from build123d import *

# Parameters (mm, degrees)
SKETCH2_W           = 3.765548925
SKETCH2_H           = 14.748929387
SKETCH2_W_2         = 4.619974481
CUT_EXTRUDE1_DEPTH  = 17.5
CHAMFER1_SIZE       = 0.353571801
CHAMFER1_SIZE_2     = 0.5
SKETCH3_R           = 3
CUT_EXTRUDE2_DEPTH  = 35
SKETCH4_R           = 3.5
SKETCH4_R_2         = 3
BOSS_EXTRUDE1_DEPTH = 15
BOSS_EXTRUDE2_DEPTH = 1
BOSS_EXTRUDE3_START = -1
SKETCH4_2_R         = 3.5
SKETCH4_2_R_2       = 3
BOSS_EXTRUDE3_DEPTH = 1
BOSS_EXTRUDE4_START = -1
BOSS_EXTRUDE4_DEPTH = 1
FILLET1_R           = 1
FILLET2_R           = 10


# Some blends are built 0.0001 mm under size
with BuildPart() as part:
    # Sketch1 → Revolve1 (revolve)
    with BuildSketch(Plane(origin=(0, 0, 0), x_dir=(0, 0, -1), z_dir=(1, 0, 0))):
        with BuildLine():
            Line((0, 3.5), (0, 0))
            Line((0, 0), (4.5, 0))
            ThreePointArc((4.5, 0), (8, 3.5), (11.5, 0))
            Line((11.5, 0), (14, 0))
            ThreePointArc((14, 0), (11.451186904, 4.908086078), (5.97023035, 5.6462408))
            Line((5.97023035, 5.6462408), (0, 3.5))
        make_face()
    revolve(axis=Axis((0, 0, 0), (0, 0, -1)))

    # Sketch2 → Cut-Extrude1 (cut, symmetric)
    with BuildSketch(Plane(origin=(0, 0, 0), x_dir=(1, 0, 0), z_dir=(0, 1, 0))):
        with Locations((-4.382774463, 6.625535306)):
            Rectangle(SKETCH2_W, SKETCH2_H)
        with Locations((4.80998724, 6.625535306)):
            Rectangle(SKETCH2_W_2, SKETCH2_H)
    extrude(amount=CUT_EXTRUDE1_DEPTH, both=True, mode=Mode.SUBTRACT)

    # Chamfer1
    # the kernel refuses this chamfer: 0.5, 0.353571801 mm, written as the material it takes off along each edge
    with BuildSketch(Plane(origin=(-2.5, 0, -8), x_dir=(0, 0, 1), z_dir=(0, 1, 0))) as chamfer1_piece_1:
        with BuildLine():
            Line((2.807242504, 0.409691525), (2.449489743 + CHAMFER1_SIZE * 0.999999998636, 0))
            Line((2.449489743 + CHAMFER1_SIZE * 0.999999998636, 0), (2.449489743, 0))
            ThreePointArc((2.449489743, 0), (2.641353047, 0.203643303), (2.807242504, 0.409691525))
        make_face()
    revolve(axis=Axis((-2.5, 0, -8), (1, 0, 0)), mode=Mode.SUBTRACT)
    with BuildSketch(Plane(origin=(2.5, 0, -8), x_dir=(0, 0, -1), z_dir=(0, 1, 0))) as chamfer1_piece_2:
        with BuildLine():
            Line((2.449489743 + CHAMFER1_SIZE_2, 0), (2.689392867, 0.260096876))
            ThreePointArc((2.689392867, 0.260096876), (2.573005025, 0.127312675), (2.449489743, 0))
            Line((2.449489743, 0), (2.449489743 + CHAMFER1_SIZE_2, 0))
        make_face()
    revolve(axis=Axis((2.5, 0, -8), (-1, 0, 0)), mode=Mode.SUBTRACT)

    # Sketch3 → Cut-Extrude2 (cut)
    with BuildSketch(Plane(origin=(2.5, 0, 0), x_dir=(0, 0, -1), z_dir=(1, 0, 0))):
        with Locations((8, 0)):
            Circle(SKETCH3_R)
    extrude(amount=-CUT_EXTRUDE2_DEPTH, mode=Mode.SUBTRACT)

    # Sketch4 → Boss-Extrude1 (add)
    with BuildSketch(Plane.XY):
        with Locations(Location((0, 0, 0), (0, 0, 135.584691403))):
            Circle(SKETCH4_R)
        with Locations(Location((0, 0, 0), (0, 0, 213.557309762))):
            Circle(SKETCH4_R_2, mode=Mode.SUBTRACT)
    extrude(amount=BOSS_EXTRUDE1_DEPTH)

    # Sketch5 → Boss-Extrude2 (add)
    with BuildSketch(Plane.XY):
        with BuildLine():
            Line((2.5, 1.658312395), (2.5, -1.658312395))
            ThreePointArc((2.5, -1.658312395), (2.872281323, -0.866025404), (3, 0))
            ThreePointArc((3, 0), (2.872281323, 0.866025404), (2.5, 1.658312395))
        make_face()
        with BuildLine():
            ThreePointArc((-2.5, -1.658312395), (0, -3), (2.5, -1.658312395))
            Line((2.5, -1.658312395), (2.5, 1.658312395))
            ThreePointArc((2.5, 1.658312395), (0, 3), (-2.5, 1.658312395))
            Line((-2.5, 1.658312395), (-2.5, -1.658312395))
        make_face()
        with BuildLine():
            ThreePointArc((-2.5, 1.658312395), (-3, 0), (-2.5, -1.658312395))
            Line((-2.5, -1.658312395), (-2.5, 1.658312395))
        make_face()
    extrude(amount=BOSS_EXTRUDE2_DEPTH)

    # Sketch4<2> → Boss-Extrude3 (add)
    with BuildSketch(Plane.XY.offset(BOSS_EXTRUDE3_START)):
        with Locations(Location((0, 0, 0), (0, 0, 135.584691403))):
            Circle(SKETCH4_2_R)
        Circle(SKETCH4_2_R_2, mode=Mode.SUBTRACT)
    extrude(amount=BOSS_EXTRUDE3_DEPTH)

    # Sketch5<4> → Boss-Extrude4 (add)
    with BuildSketch(Plane.XY.offset(BOSS_EXTRUDE4_START)):
        with BuildLine():
            Line((2.5, 1.658312395), (2.5, -1.658312395))
            ThreePointArc((2.5, -1.658312395), (2.872281323, -0.866025404), (3, 0))
            ThreePointArc((3, 0), (2.872281323, 0.866025404), (2.5, 1.658312395))
        make_face()
        with BuildLine():
            ThreePointArc((-2.5, 1.658312395), (-3, 0), (-2.5, -1.658312395))
            Line((-2.5, -1.658312395), (-2.5, 1.658312395))
        make_face()
    extrude(amount=BOSS_EXTRUDE4_DEPTH)

    # Fillet1
    fillet1_edges = [part.edges().sort_by_distance(p)[0] for p in [
        (-3.5, 0, -1),
        (3.5, 0, -1),
    ]]
    fillet(fillet1_edges, radius=FILLET1_R - 0.0001)  # a hair under: the kernel refuses the full size

    # Fillet2
    # the kernel refuses this fillet: 10 mm, written as the material it adds along each edge
    with BuildSketch(Plane(origin=(0, 0, 0), x_dir=(-0.8914706902273792, -0.453078369010837, 0), z_dir=(0.453078369010837, -0.8914706902273792, 0))) as fillet2_piece_1_section:
        with BuildLine():
            CenterArc((3.5 + FILLET2_R, -FILLET2_R * 0.174285392608), FILLET2_R, 160.226973292, 19.773026708)
            Line((3.5 + FILLET2_R * 0.0589598667305, FILLET2_R * 0.164009549087), (3.5, 0))
            Line((3.5, 0), (3.5, -FILLET2_R * 0.174285392608))
        make_face()
    fillet2_piece_1 = revolve(axis=Axis((0, 0, 0), (0, 0, -1)), revolution_arc=233.882722234, mode=Mode.PRIVATE)
    fillet2_piece_1 = split(fillet2_piece_1, bisect_by=Plane(origin=(2.5, 0, 0), z_dir=(-1, 0, 0)), keep=Keep.TOP, mode=Mode.PRIVATE)
    fillet2_piece_1 = split(fillet2_piece_1, bisect_by=Plane(origin=(-2.5, 0, 0), z_dir=(1, 0, 0)), keep=Keep.TOP, mode=Mode.PRIVATE)
    add(fillet2_piece_1)
    with BuildSketch(Plane(origin=(0, 0, 0), x_dir=(0.8914706902273793, 0.4530783690108364, 0), z_dir=(-0.4530783690108364, 0.8914706902273793, 0))) as fillet2_piece_2_section:
        with BuildLine():
            CenterArc((3.5 + FILLET2_R, -FILLET2_R * 0.174285392608), FILLET2_R, 160.226973292, 19.773026708)
            Line((3.5 + FILLET2_R * 0.0589598667305, FILLET2_R * 0.164009549087), (3.5, 0))
            Line((3.5, 0), (3.5, -FILLET2_R * 0.174285392608))
        make_face()
    fillet2_piece_2 = revolve(axis=Axis((0, 0, 0), (0, 0, -1)), revolution_arc=233.882722234, mode=Mode.PRIVATE)
    fillet2_piece_2 = split(fillet2_piece_2, bisect_by=Plane(origin=(2.5, 0, 0), z_dir=(-1, 0, 0)), keep=Keep.TOP, mode=Mode.PRIVATE)
    fillet2_piece_2 = split(fillet2_piece_2, bisect_by=Plane(origin=(-2.5, 0, 0), z_dir=(1, 0, 0)), keep=Keep.TOP, mode=Mode.PRIVATE)
    add(fillet2_piece_2)


solid = part.part
Here's how the part is built. I have some questions about the finished solid (model axes, mm). A direction names the side the tool comes from. Coordinates: 2 decimals unless noted, no trailing zeros. Write each loop counter-clockwise with the first axis right and the second up, starting at its lowest first coordinate (ties: lowest second). Pieces come first, ordered by that corner, then holes.
Item 1: Will these pins go through, and if not, where does the flat tip stop? pin 1 (4 mm diameter, centred on x = 3, z = 4.5, fed in from +Y); pin 2 (2 mm diameter, centred on y = 0.5, z = 2.5, fed in from -X); pin 3 (3 mm diameter, centred on y = 4, z = -0.5, fed in from -X); pin 4 (5 mm diameter, centred on y = 0, z = -8, fed in from +X).
Item 2: On a 3-axis mill with a long thin cutter (end or side, diameter ignored), from which of +Z, -Z, +X, -X, +Y, -Y can I reach the whole of each face in a straight line? I mean faces 1 (the cylindrical face through (-2.15, -1.15, -10.77)), 2 (the cylindrical face through (1.02, 3.35, 7.39)). Say none if no direction works.
Item 3: I want a section at C-C on z = -3. Write out the boundary of the cut face in (x, y).
Item 4: If we mould it in two halves opening along Y, with no side actions, what happens to faces 3 (the flat face through (0, 0, 1)), 4 (the flat face through (2.5, 2.3, -5.7)), 5 (the conical face through (-0.045, 4.857, -3.775))? For each: +Y half, -Y half, draft (parallel to the pull), parting line (faces both ways), or undercut.
Item 5: I want a section at B-B on x = 0. Write out the boundary of the cut face in (y, z).
Item 6: I want a section at A-A on z = -8. Write out the boundary of the cut face in (x, y), and give its area (3 significant figures).
Item 7: If I drill on line 1 (Y direction, x = 0, z = 6); line 2 (X direction, y = -2.75, z = -2.5); line 3 (Z direction, x = 2.15, y = 0), over which ranges is the centre line in solid material (lowest first)?
Findings below:
1. pin 1: stops at y = 3.35
1. pin 2: stops at x = -3.5
1. pin 3: stops at x = -2.5
1. pin 4: passes through
2. face 1: +X, -X
2. face 2: +Z
3. outline: (-2.5, -3.84) arc R4.58 ccw to (2.5, -3.84) - (2.5, 3.84) arc R4.58 ccw to (-2.5, 3.84) - close
4. face 3: undercut
4. face 4: draft
4. face 5: +Y half
5. outline: (-5.65, -5.97) arc R6 ccw (long way) to (5.65, -5.97) - (4.09, -1.64) arc R10 cw to (3.5, 1.74) - (3.5, 15) - (3, 15) - (3, 1) - (-3, 1) - (-3, 15) - (-3.5, 15) - (-3.5, 1.74) arc R10 cw to (-4.09, -1.64) - close; hole circle Ø7 at (0, -8)
6. outline: (-2.5, -5.45) arc R6 ccw to (2.5, -5.45) - (2.5, -3) - (1.8, -3) arc R3.5 cw to (-1.8, -3) - (-2.5, -3) - close; (-2.5, 3) - (-1.8, 3) arc R3.5 cw to (1.8, 3) - (2.5, 3) - (2.5, 5.45) arc R6 ccw to (-2.5, 5.45) - close
6. area: 25.8 mm2
7. line 1: y = -3.5 to -3, 3 to 3.5
7. line 2: x = -2.5 to 2.5
7. line 3: z = -13.6 to -11, -5 to 1
